```python
from build123d import *

# Parameters (mm, degrees)
BOSS_EXTRUDE3_DEPTH   = 8
BOSS_EXTRUDE3_2_DEPTH = 8
SKETCH4_W             = 14
SKETCH4_H             = 17.5
BOSS_EXTRUDE4_DEPTH   = 2
FILLET3_R             = 3
MIRROR2_START         = -2
MIRROR2_DEPTH         = 10
MIRROR2_2_DEPTH       = 2
CHAMFER1_SIZE         = 2
FILLET4_R             = 9
FILLET5_R             = 2


# Read off the part's stored shape, not the designer's step: Mirror2
with BuildPart() as part:
    # Sketch3 → Boss-Extrude3 (new body)
    with BuildSketch(Plane(origin=(0, 0, 0), x_dir=(1, 0, 0), z_dir=(0, 1, 0))):
        with BuildLine():
            Line((-1.7, -8.75), (7, -8.75))
            Line((7, -8.75), (7, 8.75))
            Line((7, 8.75), (-7, 8.75))
            Line((-7, 8.75), (-7, -8.75))
            Line((-7, -8.75), (-4, -8.75))
            Line((-4, -8.75), (-4, 3.25))
            ThreePointArc((-4, 3.25), (1, 8.25), (6, 3.25))
            Line((6, 3.25), (6, 2.25))
            ThreePointArc((6, 2.25), (3.397915762, -2.137482194), (-1.7, -1.958325083))
            Line((-1.7, -1.958325083), (-1.7, -8.75))
        make_face()
    extrude(amount=BOSS_EXTRUDE3_DEPTH)



with BuildPart() as body_2:
    # Sketch3 → Boss-Extrude3 2 (new body)
    with BuildSketch(Plane(origin=(0, 0, 0), x_dir=(1, 0, 0), z_dir=(0, 1, 0))):
        with BuildLine():
            ThreePointArc((-2.2, 2.25), (1, -0.95), (4.2, 2.25))
            Line((4.2, 2.25), (4.2, 3.25))
            ThreePointArc((4.2, 3.25), (1, 6.45), (-2.2, 3.25))
            Line((-2.2, 3.25), (-2.2, 2.25))
        make_face()
    extrude(amount=BOSS_EXTRUDE3_2_DEPTH)


with BuildPart() as part_1:
    add(part.part)

    add(body_2.part)  # Boss-Extrude4 merges body 2
    # Sketch4 → Boss-Extrude4 (add)
    with BuildSketch(Plane(origin=(0, 0, 0), x_dir=(-1, 0, 0), z_dir=(0, -1, 0))):
        Rectangle(SKETCH4_W, SKETCH4_H)
    extrude(amount=BOSS_EXTRUDE4_DEPTH)

    # Fillet3
    fillet3_edges = [part_1.edges().sort_by_distance(p)[0] for p in [
        (-1.7, 4, 1.958325083),
    ]]
    fillet(fillet3_edges, radius=FILLET3_R)

    # Mirror2 outline → Mirror2 (add)
    with BuildSketch(Plane(origin=(0, 0, 0), x_dir=(1, 0, 0), z_dir=(0, 1, 0)).offset(MIRROR2_START)):
        with BuildLine():
            ThreePointArc((1.1875, 20.246483138), (4.601215073, 18.718609231), (6, 15.25))
            Line((6, 15.25), (6, 14.25))
            ThreePointArc((6, 14.25), (1, 9.25), (-4, 14.25))
            Line((-4, 14.25), (-4, 26.25))
            Line((-4, 26.25), (-7, 26.25))
            Line((-7, 26.25), (-7, 8.75))
            Line((-7, 8.75), (7, 8.75))
            Line((7, 8.75), (7, 26.25))
            Line((7, 26.25), (-1.7, 26.25))
            Line((-1.7, 26.25), (-1.7, 23.244373021))
            ThreePointArc((-1.7, 23.244373021), (-0.860729044, 21.163207482), (1.1875, 20.246483138))
        make_face()
        with BuildLine():
            ThreePointArc((-2.2, 14.25), (1, 11.05), (4.2, 14.25))
            Line((4.2, 14.25), (4.2, 15.25))
            ThreePointArc((4.2, 15.25), (1, 18.45), (-2.2, 15.25))
            Line((-2.2, 15.25), (-2.2, 14.25))
        make_face()
    extrude(amount=MIRROR2_DEPTH)

    # Mirror2 2 outline → Mirror2 2 (add)
    with BuildSketch(Plane(origin=(0, 0, 0), x_dir=(1, 0, 0), z_dir=(0, 1, 0)).offset(MIRROR2_START)):
        with BuildLine():
            Line((6, 14.25), (6, 15.25))
            ThreePointArc((6, 15.25), (4.601215073, 18.718609231), (1.1875, 20.246483138))
            ThreePointArc((1.1875, 20.246483138), (-0.860729044, 21.163207482), (-1.7, 23.244373021))
            Line((-1.7, 23.244373021), (-1.7, 26.25))
            Line((-1.7, 26.25), (-4, 26.25))
            Line((-4, 26.25), (-4, 14.25))
            ThreePointArc((-4, 14.25), (1, 9.25), (6, 14.25))
        make_face()
        with BuildLine():
            Line((4.2, 15.25), (4.2, 14.25))
            ThreePointArc((4.2, 14.25), (1, 11.05), (-2.2, 14.25))
            Line((-2.2, 14.25), (-2.2, 15.25))
            ThreePointArc((-2.2, 15.25), (1, 18.45), (4.2, 15.25))
        make_face(mode=Mode.SUBTRACT)
    extrude(amount=MIRROR2_2_DEPTH)

    # Chamfer1
    # the kernel refuses this chamfer: 2 mm, written as the material it adds along each edge
    with BuildSketch(Plane(origin=(1, 0, -14.25), x_dir=(1, 0, 0), z_dir=(0, 0, -1))) as chamfer1_piece_1:
        Polygon((3.2 + CHAMFER1_SIZE, 0), (3.2, -CHAMFER1_SIZE), (3.2, 0), align=None)
    revolve(axis=Axis((1, 0, -14.25), (0, -1, 0)), revolution_arc=180)
    with BuildSketch(Plane(origin=(-2.2, 0, -14.25), x_dir=(-0.9996219169112968, -0.027495876610586365, 0), z_dir=(0, 0, -1)), Plane(origin=(4.2, 0, -15.25), x_dir=(0.9996219169112968, -0.027495876610586365, 0), z_dir=(0, 0, 1))) as chamfer1_piece_2:
        Polygon((CHAMFER1_SIZE * 0.999621916911, CHAMFER1_SIZE * 0.0274958766106), (-CHAMFER1_SIZE * 0.0274958766106, CHAMFER1_SIZE * 0.999621916911), (0, 0), align=None)
    extrude(amount=1)
    with BuildSketch(Plane(origin=(1, 0, -15.25), x_dir=(-1, 0, 0), z_dir=(0, 0, 1))) as chamfer1_piece_3:
        Polygon((3.2 + CHAMFER1_SIZE, 0), (3.2, -CHAMFER1_SIZE), (3.2, 0), align=None)
    revolve(axis=Axis((1, 0, -15.25), (0, -1, 0)), revolution_arc=180)
    with BuildSketch(Plane(origin=(1, 0, -3.25), x_dir=(1, 0, 0), z_dir=(0, 0, 1))) as chamfer1_piece_4:
        Polygon((3.2 + CHAMFER1_SIZE, 0), (3.2, CHAMFER1_SIZE), (3.2, 0), align=None)
    revolve(axis=Axis((1, 0, -3.25), (0, 1, 0)), revolution_arc=180)
    with BuildSketch(Plane(origin=(-2.2, 0, -3.25), x_dir=(-0.9996219169112968, -0.027495876610586365, 0), z_dir=(0, 0, 1)), Plane(origin=(4.2, 0, -2.25), x_dir=(0.9996219169112968, -0.027495876610586365, 0), z_dir=(0, 0, -1))) as chamfer1_piece_5:
        Polygon((CHAMFER1_SIZE * 0.999621916911, -CHAMFER1_SIZE * 0.0274958766106), (-CHAMFER1_SIZE * 0.0274958766106, -CHAMFER1_SIZE * 0.999621916911), (0, 0), align=None)
    extrude(amount=1)
    with BuildSketch(Plane(origin=(1, 0, -2.25), x_dir=(-1, 0, 0), z_dir=(0, 0, -1))) as chamfer1_piece_6:
        Polygon((3.2 + CHAMFER1_SIZE, 0), (3.2, CHAMFER1_SIZE), (3.2, 0), align=None)
    revolve(axis=Axis((1, 0, -2.25), (0, 1, 0)), revolution_arc=180)

    # Fillet4
    fillet4_edges = [part_1.edges().sort_by_distance(p)[0] for p in [
        (7, 3, 8.75),
        (7, 3, -26.25),
    ]]
    fillet(fillet4_edges, radius=FILLET4_R)

    # Fillet5
    fillet5_edges = [part_1.edges().sort_by_distance(p)[0] for p in [
        (-7, 3, 8.75),
        (-7, 3, -26.25),
    ]]
    fillet(fillet5_edges, radius=FILLET5_R)


solid = part_1.part
```
For this review, take the finished solid that the model builds, in its own axes (mm). A direction names the side the tool comes from. Give positions to 0.01 mm unless a question says otherwise; leave off trailing zeros. Loops run counter-clockwise (first coordinate to the right, second up) from the corner with the lowest first, then second, coordinate; pieces in that order, holes last. Notation, with made-up numbers: M -37,6 L -15,6 A27 ccw -15,43 Z; hole C 80.25,89 d6. An arc over 180 degrees is marked long. One line per item, written item: value. Start each with the question number.
Q1. Draft analysis for pull direction X (two halves, no side actions). For faces 1 (the face through (-4, 4, -20)), 2 (the face through (4.294, 2.93, 6.184)), state which applies: released by +X, released by -X, zero draft, split by the parting line, or undercut.
Q2. For L1, parallel to Z at x = 2.75, y = 3.75; L2, parallel to Z at x = 1, y = 4.75; L3, parallel to X at y = 5, z = -0.5, list the stretches that pass through material, from the lowest coordinate up.
Q3. Add section B-B (y = -1.5). Give the boundary of the cut face in (x, z), and give its area (3 significant figures).
Q4. Add section A-A (y = 3). Count the separate pieces of the cut face and the enclosed holes in it, and give its area (3 significant figures).
Q5. Clearance check with flat-ended pins moving along their axes: pin 1 Ø1.3 at (x, z) = (-1.5, 2.5) entering from +Y; pin 2 Ø2.5 at (y, z) = (2.5, 3) entering from +X; pin 3 Ø3 at (x, y) = (1.5, 6) entering from +Z. State where each tip first meets the part, or that it passes through.
Q6. Machinability: for faces 3 (the face through (-2.2, 5, -15)), 4 (the face through (-0.883, 3.944, -21.187)), 5 (the face through (-2.2, 5, -3)), which of the approach directions +Z, -Z, +X, -X, +Y, -Y give a long, thin tool a straight path to every point of the face, cutting with its end or side? Answer none if there is none.
Reply:
1. face 1: undercut
1. face 2: released by +X
2. L1: -24.89 to -19.93, -17.93 to -11.57, -9.57 to -7.93, -5.93 to 0.43, 2.43 to 7.39
2. L2: -25.74 to -20.26, -18.45 to -11.05, -9.25 to -8.25, -6.45 to 0.95, 2.76 to 8.24
2. L3: -7 to -4, -1.68 to 3.68, 5.68 to 7
3. outline: M -7,-24.25 A2 ccw -5,-26.25 L -2,-26.25 A9 ccw 7,-17.25 L 7,-0.25 A9 ccw -2,8.75 L -5,8.75 A2 ccw -7,6.75 Z
3. area: 454 mm²
4. separate pieces: 3
4. enclosed holes: 0
4. area: 311 mm²
5. pin 1: y = 0.48
5. pin 2: x = 6.77
5. pin 3: z = 8.52
6. face 3: -Z, +Y
6. face 4: +Y
6. face 5: +Z, +Y
